from build123d import *

# Parameters (mm, degrees)
EXTRUDE_1_DEPTH      = 5
SKETCH_4_W           = 45
SKETCH_4_H           = 30
CUT_EXTRUDE_3_DEPTH  = 5
SKETCH_5_W           = 75
SKETCH_5_H           = 160
CUT_EXTRUDE_4_DEPTH  = 5
CUT_EXTRUDE_5_REACH  = 335.054
SKETCH_6_R           = 1.5
CUT_EXTRUDE_9_REACH  = 335.054
SKETCH_9_R           = 1.5
SKETCH_11_R          = 1.5
CUT_EXTRUDE_10_DEPTH = 5


with BuildPart() as part:
    # 草图1 → 凸台-拉伸1 (new body)
    with BuildSketch(Plane(origin=(0, 0, 0), x_dir=(1, 0, 0), z_dir=(0, 1, 0))):
        with BuildLine():
            Line((10, 0), (240, 0))
            ThreePointArc((240, 0), (247.071067812, -2.928932188), (250, -10))
            Line((250, -10), (250, -210))
            ThreePointArc((250, -210), (247.071067812, -217.071067812), (240, -220))
            Line((240, -220), (10, -220))
            ThreePointArc((10, -220), (2.928932188, -217.071067812), (0, -210))
            Line((0, -210), (0, -10))
            ThreePointArc((0, -10), (2.928932188, -2.928932188), (10, 0))
        make_face()
    extrude(amount=EXTRUDE_1_DEPTH)

    # 草图4 → 切除-拉伸3 (cut)
    with BuildSketch(Plane.XZ):
        with Locations((192.5, 49.475)):
            Rectangle(SKETCH_4_W, SKETCH_4_H)
        with Locations((57.5, 49.475)):
            Rectangle(SKETCH_4_W, SKETCH_4_H)
    extrude(amount=-CUT_EXTRUDE_3_DEPTH, mode=Mode.SUBTRACT)

    # 草图5 → 切除-拉伸4 (cut)
    with BuildSketch(Plane.XZ):
        with Locations((125, 140)):
            Rectangle(SKETCH_5_W, SKETCH_5_H)
    extrude(amount=-CUT_EXTRUDE_4_DEPTH, mode=Mode.SUBTRACT)

    # 草图6 → 切除-拉伸5 (cut, up to next)
    with BuildSketch(Plane.XZ, mode=Mode.PRIVATE) as cut_extrude_5_sk1:
        with Locations(Location((72.5, 200, 0), (0, 0, 270))):
            Circle(SKETCH_6_R)
    cut_extrude_5_tool1 = extrude(cut_extrude_5_sk1.sketch, amount=-CUT_EXTRUDE_5_REACH, mode=Mode.PRIVATE) & part.part
    # 草图6 → 切除-拉伸5 (cut, up to next)
    with BuildSketch(Plane.XZ, mode=Mode.PRIVATE) as cut_extrude_5_sk2:
        with Locations(Location((177.5, 200, 0), (0, 0, 90))):
            Circle(SKETCH_6_R)
    cut_extrude_5_tool2 = extrude(cut_extrude_5_sk2.sketch, amount=-CUT_EXTRUDE_5_REACH, mode=Mode.PRIVATE) & part.part
    add(cut_extrude_5_tool1.solids().sort_by_distance((72.5, 0, 200))[0], mode=Mode.SUBTRACT)
    add(cut_extrude_5_tool2.solids().sort_by_distance((177.5, 0, 200))[0], mode=Mode.SUBTRACT)

    # 草图9 → 切除-拉伸9 (cut, up to next)
    with BuildSketch(Plane.XZ, mode=Mode.PRIVATE) as cut_extrude_9_sk1:
        with Locations(Location((77.5, 15, 0), (0, 0, 270))):
            Circle(SKETCH_9_R)
    cut_extrude_9_tool1 = extrude(cut_extrude_9_sk1.sketch, amount=-CUT_EXTRUDE_9_REACH, mode=Mode.PRIVATE) & part.part
    # 草图9 → 切除-拉伸9 (cut, up to next)
    with BuildSketch(Plane.XZ, mode=Mode.PRIVATE) as cut_extrude_9_sk2:
        with Locations(Location((10, 210, 0), (0, 0, 270))):
            Circle(SKETCH_9_R)
    cut_extrude_9_tool2 = extrude(cut_extrude_9_sk2.sketch, amount=-CUT_EXTRUDE_9_REACH, mode=Mode.PRIVATE) & part.part
    # 草图9 → 切除-拉伸9 (cut, up to next)
    with BuildSketch(Plane.XZ, mode=Mode.PRIVATE) as cut_extrude_9_sk3:
        with Locations(Location((240, 210, 0), (0, 0, 90))):
            Circle(SKETCH_9_R)
    cut_extrude_9_tool3 = extrude(cut_extrude_9_sk3.sketch, amount=-CUT_EXTRUDE_9_REACH, mode=Mode.PRIVATE) & part.part
    # 草图9 → 切除-拉伸9 (cut, up to next)
    with BuildSketch(Plane.XZ, mode=Mode.PRIVATE) as cut_extrude_9_sk4:
        with Locations(Location((172.5, 15, 0), (0, 0, 90))):
            Circle(SKETCH_9_R)
    cut_extrude_9_tool4 = extrude(cut_extrude_9_sk4.sketch, amount=-CUT_EXTRUDE_9_REACH, mode=Mode.PRIVATE) & part.part
    add(cut_extrude_9_tool1.solids().sort_by_distance((77.5, 0, 15))[0], mode=Mode.SUBTRACT)
    add(cut_extrude_9_tool2.solids().sort_by_distance((10, 0, 210))[0], mode=Mode.SUBTRACT)
    add(cut_extrude_9_tool3.solids().sort_by_distance((240, 0, 210))[0], mode=Mode.SUBTRACT)
    add(cut_extrude_9_tool4.solids().sort_by_distance((172.5, 0, 15))[0], mode=Mode.SUBTRACT)

    # 草图11 → 切除-拉伸10 (cut)
    with BuildSketch(Plane.XZ):
        with Locations(Location((240, 180, 0), (0, 0, 270))):
            Circle(SKETCH_11_R)
        with Locations(Location((240, 140, 0), (0, 0, 270))):
            Circle(SKETCH_11_R)
        with Locations(Location((10, 143.83552588, 0), (0, 0, 270))):
            Circle(SKETCH_11_R)
        with Locations(Location((10, 183.83552588, 0), (0, 0, 270))):
            Circle(SKETCH_11_R)
    extrude(amount=-CUT_EXTRUDE_10_DEPTH, mode=Mode.SUBTRACT)


solid = part.part
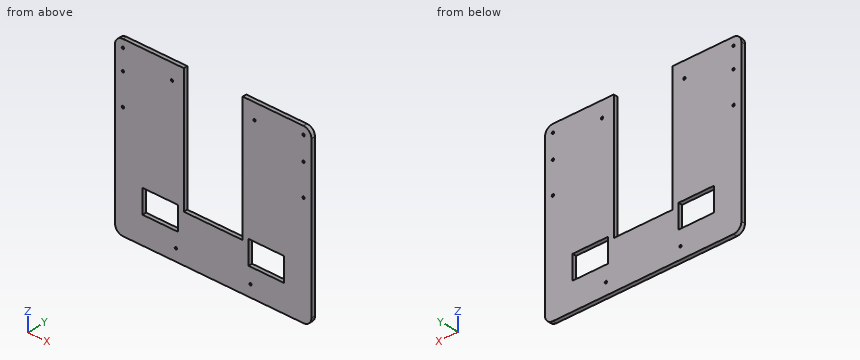
Source: CAD feature listing. Evaluate the final solid. Frame: model axes, mm. Give positions to 0.01 mm unless a question says otherwise; leave off trailing zeros. Order: outer loops, then holes, each group sorted by start corner. A loop starts at its lowest first (then second) coordinate and runs counter-clockwise, first axis right, second up. Notation, with made-up numbers: (76.25, 30) -> (110.25, 30) arc R24 ccw to (110.25, 53) -> close; hole circle Ø1 at (-27, 89.25). An arc over 180 degrees is marked (long way). Write item = value, one per line.
Item 1: Section query A-A (x = 62). Output: boundary loops of the cut face in (y, z) (3 decimals), then the cut area to 3 significant figures.
Check result:
outline = (0, 0) -> (5, 0) -> (5, 34.475) -> (0, 34.475) -> close; (0, 64.475) -> (5, 64.475) -> (5, 220) -> (0, 220) -> close
area = 950 mm²
Item 2: Contact query for flat-ended pins moving along their axis: pin 1 (2 mm diameter, centred on x = 71, z = 105.5, fed in from -Y); pin 2 (2.5 mm diameter, centred on x = 240, z = 180, fed in from -Y). Output: stop coordinate, or through.
Check result:
pin_1 = 0
pin_2 = through
Item 3: Ray query, probe 1 along X at (y, z) = (2.5, 15); probe 2 along X at (y, z) = (1.5, 38); probe 3 along Z at (x, y) = (240, 3.35). Return the intervals inside material, ascending.
Check result:
probe_1 = 0 to 76, 79 to 171, 174 to 250
probe_2 = 0 to 35, 80 to 170, 215 to 250
probe_3 = 0 to 138.5, 141.5 to 178.5, 181.5 to 208.5, 211.5 to 220
Item 4: Section query B-B (z = 92). Output: boundary loops of the cut face in (x, y).
Check result:
outline = (0, 0) -> (87.5, 0) -> (87.5, 5) -> (0, 5) -> close; (162.5, 0) -> (250, 0) -> (250, 5) -> (162.5, 5) -> close
Item 5: Section query C-C (y = 1.8). State how many separate pieces and enclosed holes the cut face has, then the cut area to 3 significant figures.
Check result:
separate_pieces = 1
enclosed_holes = 12
area = 40,100 mm²
Item 6: Section query D-D (x = 94). Output: boundary loops of the cut face in (y, z), then the cut area to 3 significant figures.
Check result:
outline = (0, 0) -> (5, 0) -> (5, 60) -> (0, 60) -> close
area = 300 mm²
